from build123d import *

# Parameters (mm, degrees)
SKETCH1_R           = 2.1
SKETCH1_R_2         = 5
BOSS_EXTRUDE2_DEPTH = 8
FILLET1_R           = 2


with BuildPart() as part:
    # Sketch1 → Boss-Extrude2 (new body)
    with BuildSketch(Plane(origin=(0, 0, 0), x_dir=(1, 0, 0), z_dir=(0, 1, 0))):
        with BuildLine():
            Line((0, 46.1), (0, 38.1))
            ThreePointArc((0, 38.1), (38.1, 0), (0, -38.1))
            Line((0, -38.1), (0, -73.400550657))
            ThreePointArc((0, -73.400550657), (25.844530788, -91.377376201), (8, -65.441325051))
            Line((8, -65.441325051), (8, -45.400550657))
            ThreePointArc((8, -45.400550657), (45.924804764, 4.015259312), (0, 46.1))
        make_face()
        with Locations(Location((22.559764633, -72.034799208, 0), (0, 0, 270))):
            Circle(SKETCH1_R, mode=Mode.SUBTRACT)
        with Locations(Location((22.559764633, -88.034799208, 0), (0, 0, 270))):
            Circle(SKETCH1_R, mode=Mode.SUBTRACT)
        with Locations(Location((6.559764633, -88.034799208, 0), (0, 0, 270))):
            Circle(SKETCH1_R, mode=Mode.SUBTRACT)
        with Locations(Location((6.559764633, -72.034799208, 0), (0, 0, 270))):
            Circle(SKETCH1_R, mode=Mode.SUBTRACT)
        with Locations(Location((14.559764633, -80.034799208, 0), (0, 0, 270))):
            Circle(SKETCH1_R_2, mode=Mode.SUBTRACT)
    extrude(amount=BOSS_EXTRUDE2_DEPTH)

    # Fillet1
    fillet1_edges = [part.edges().sort_by_distance(p)[0] for p in [
        (0, 4, 38.1),
        (0, 4, -38.1),
        (0, 4, -46.1),
        (8, 4, 45.400550657),
        (8, 4, 65.441325051),
        (0, 4, 73.400550657),
    ]]
    fillet(fillet1_edges, radius=FILLET1_R)


solid = part.part
Read the model definition and answer for the solid it produces. Units are mm, in the model's axes. A direction names the side the tool comes from. Round coordinates to 2 decimals unless told otherwise and drop trailing zeros. Write each loop counter-clockwise with the first axis right and the second up, starting at its lowest first coordinate (ties: lowest second). Pieces come first, ordered by that corner, then holes. Notation, with made-up numbers: M 46.5,-36.5 L 56.5,-36.5 A25 cw 56.5,2.5 Z; hole C 14,45 d11. An arc over 180 degrees is marked long. Use a Markdown table: item, result.
1) Flat-ended cylindrical pins translate along their axes: pin 1 (3.5 mm diameter, centred on x = 6.56, z = 88.03, fed in from -Y); pin 2 (3 mm diameter, centred on y = 4, z = -41, fed in from -X); pin 3 (4 mm diameter, centred on x = 26.5, y = 5.5, fed in from +Z); pin 4 (1 mm diameter, centred on x = 36, y = 7, fed in from +Z). Find the tip coordinate at first contact, or state that the pin passes through.
Answers follow:
| item | result |
|---|---|
| pin 1 | passes through |
| pin 2 | stops at x = 0 |
| pin 3 | stops at z = 92.57 |
| pin 4 | stops at z = 29.41 |
2) The part is cut by section A-A (y = 2.25). Write down the section's boundary in (x, z), plus the area to 3 significant figures.
Answers follow:
| item | result |
|---|---|
| outline | M -0.16,73.76 A2 cw 0,72.98 L 0,40.05 A2 ccw 1.9,38.05 A38.1 cw 1.9,-38.05 A2 ccw 0,-40.05 L 0,-44.05 A2 ccw 2.09,-46.05 A46.1 ccw 9.58,45.09 A2 cw 8,47.05 L 8,62.62 A2 cw 10.51,64.56 A16 ccw long Z; hole C 6.56,72.03 d4.2; hole C 6.56,88.03 d4.2; hole C 14.56,80.03 d10; hole C 22.56,72.03 d4.2; hole C 22.56,88.03 d4.2 |
| area | 1,910 mm2 |
3) Straight lines are drawn through the part: line 1 along Z through (x, y) = (12, 2); line 2 along Z through (x, y) = (12.5, 6); line 3 along X through (y, z) = (3.5, 72.5). For each, find the intervals that lie inside material, in ascending order. Write a range as [from, to].
Answers follow:
| item | result |
|---|---|
| line 1 | z = [-44.51, -36.16], [36.16, 44.51], [64.24, 75.74], [84.33, 95.83] |
| line 2 | z = [-44.37, -35.99], [35.99, 44.37], [64.17, 75.48], [84.59, 95.9] |
| line 3 | x = [0, 4.51], [8.61, 20.51], [24.61, 28.67] |
4) A tool of negligible diameter and unlimited length cuts with its end or side. For faces 1 (the cylindrical face through (38.09, 3.94, -0.81)), 2 (the flat face through (8, 4, 55)), 3 (the cylindrical face through (8.76, 4.06, 64.19)), 4 (the flat face through (24, 0, 30)), 5 (the flat face through (0, 4, -42)), from which of +Z, -Z, +X, -X, +Y, -Y can it reach the whole face along a straight path? Write none if from no direction.
Answers follow:
| item | result |
|---|---|
| face 1 | -X, +Y, -Y |
| face 2 | +X, +Y, -Y |
| face 3 | +Y, -Y |
| face 4 | +Z, -Z, +X, -X, -Y |
| face 5 | -Z, -X, +Y, -Y |
5) For a pull along X with two mould halves and no side action, classify faces 6 (the flat face through (24, 8, 30)), 7 (the cylindrical face through (14.78, 3.94, 75.04)), 8 (the flat face through (0, 4, 56)) as pulls with the +X half, pulls with the -X half, needs draft (parallel to the pull), parting line crosses it, or undercut.
Answers follow:
| item | result |
|---|---|
| face 6 | needs draft |
| face 7 | undercut |
| face 8 | pulls with the -X half |
6) The part is cut by section B-B (x = 13). Write down the section's boundary in (y, z), plus the area to 3 significant figures.
Answers follow:
| item | result |
|---|---|
| outline | M 0,-44.23 L 8,-44.23 L 8,-35.81 L 0,-35.81 Z; M 0,35.81 L 8,35.81 L 8,44.23 L 0,44.23 Z; M 0,64.11 L 8,64.11 L 8,75.28 L 0,75.28 Z; M 0,84.79 L 8,84.79 L 8,95.96 L 0,95.96 Z |
| area | 313 mm2 |
7) The part is cut by section C-C (z = 0). Write down the section's boundary in (x, y).
Answers follow:
| item | result |
|---|---|
| outline | M 38.1,0 L 46.1,0 L 46.1,8 L 38.1,8 Z |
8) The part is cut by section D-D (z = -34). Write down the section's boundary in (x, y).
Answers follow:
| item | result |
|---|---|
| outline | M 17.19,0 L 31.13,0 L 31.13,8 L 17.19,8 Z |
